```python
from build123d import *

# Parameters (mm, degrees)
F0_R      = 8.5
F1_DEPTH  = 9.5
F3_W      = 16
F3_H      = 14
F4_DEPTH  = 1
F5_W      = 3
F5_H      = 0.5
F6_DEPTH  = 4
F7_R      = 3.5
F8_DEPTH  = 6.5
F9_R      = 3
F10_DEPTH = 13.5
F12_DEPTH = 2


with BuildPart() as f1:
    # F0 (on Front) → F1 (new body)
    with BuildSketch(Plane.XZ):
        Circle(F0_R)
    extrude(amount=-F1_DEPTH)

    # F3 (on offset) → F4 (join)
    with BuildSketch(Plane.XZ.offset(-3.8)):
        with Locations((0, -6)):
            Rectangle(F3_W, F3_H)
    extrude(amount=F4_DEPTH)

    # F5 (on face) → F6 (join)
    with BuildSketch(Plane(origin=(0, 3.8, 0), x_dir=(-1, 0, 0), z_dir=(0, 1, 0))):
        with Locations((0, -12.75)):
            Rectangle(F5_W, F5_H)
        with Locations((-5, -12.75)):
            Rectangle(F5_W, F5_H)
        with Locations((5, -12.75)):
            Rectangle(F5_W, F5_H)
    extrude(amount=F6_DEPTH)

    # F7 (on face) → F8 (join)
    with BuildSketch(Plane.XZ):
        Circle(F7_R)
    extrude(amount=F8_DEPTH)

    # F9 (on face) → F10 (join)
    with BuildSketch(Plane.XZ.offset(6.5)):
        Circle(F9_R)
    extrude(amount=F10_DEPTH)

    # F11 (on face) → F12 (join)
    with BuildSketch(Plane.XZ.offset(6.5)):
        Polygon((5, -2.886751), (5, 2.886751), (0, 5.773503), (-5, 2.886751), (-5, -2.886751), (0, -5.773503), align=None)
    extrude(amount=-F12_DEPTH)


solid = f1.part
```
The model under review builds one solid part; all positions refer to its coordinate system, in mm. A direction names the side the tool comes from. Round coordinates to 2 decimals unless told otherwise and drop trailing zeros. Write each loop counter-clockwise with the first axis right and the second up, starting at its lowest first coordinate (ties: lowest second). Pieces come first, ordered by that corner, then holes. Notation, with made-up numbers: M 22,82 L 76,82 A22 ccw 76,91 Z; hole C 37.5,85.25 d8. An arc over 180 degrees is marked long. Use CSV: the item, a comma, the result in double quotes. Start each with the question number.
(1) For line 1 along Y through (x, z) = (-4.25, 0.5); line 2 along Y through (x, z) = (-5.25, 5.5); line 3 along Y through (x, z) = (6, -9.75), list the stretches that pass through material, from the lowest coordinate up.
(2) Clearance check with flat-ended pins moving along their axes: P1, Ø0.6, axis at y = 5.5, z = -12.5, coming from the +X side; P2, Ø5, axis at x = 0.5, z = -9.5, coming from the -Y side; P3, Ø1.5, axis at x = -6, y = -0.5, coming from the +Z side. State where each tip first meets the part, or that it passes through.
(3) We need section A-A, the plane y = -5. State the section outline as (x, z) points.
(4) We need section C-C, the plane z = 0. State the section outline as (x, y) points, then the cut area to 3 significant figures.
(5) The part is to be moulded in two halves that separate along Z. For faces 6 (the face through (-5, -6, 0)), 7 (the face through (0, 3.8, -10)), 8 (the face through (-3, -13, 0)), say which applies: +Z half, -Z half, draft (parallel to the pull), parting line (faces both ways), or undercut.
(6) We need section D-D, the plane x = 4.5. State the section outline as (y, z) points, then the cut area to 3 significant figures.
(7) Tool access review of faces 1 (the face through (-2.535, -5.514, -4.31)), 2 (the face through (3.233, -2.218, -1.341)), 3 (the face through (0, 2.8, -10)), 4 (the face through (5, -6, 0)), 5 (the face through (-5, 6, -12.5)): name each direction out of +Z, -Z, +X, -X, +Y, -Y from which nothing blocks a thin tool from reaching the whole face with its end or side.
(8) We need section B-B, the plane x = 7.5. State the section outline as (y, z) points, then the cut area to 3 significant figures.
Findings:
1,line 1,"-6.5 to -4.5, 0 to 9.5"
1,line 2,"0 to 9.5"
1,line 3,"2.8 to 3.8"
2,P1,"x = 6.5"
2,P2,"y = 0"
2,P3,"z = 6.53"
3,outline,"M -5,-2.89 L 0,-5.77 L 5,-2.89 L 5,2.89 L 0,5.77 L -5,2.89 Z"
4,outline,"M -8.5,0 L -3.5,0 L -3.5,-4.5 L -5,-4.5 L -5,-6.5 L -3,-6.5 L -3,-20 L 3,-20 L 3,-6.5 L 5,-6.5 L 5,-4.5 L 3.5,-4.5 L 3.5,0 L 8.5,0 L 8.5,9.5 L -8.5,9.5 Z"
4,area,"294 mm^2"
5,face 6,"draft"
5,face 7,"undercut"
5,face 8,"parting line"
6,outline,"M -6.5,-3.18 L -4.5,-3.18 L -4.5,3.18 L -6.5,3.18 Z; M 0,-7.21 L 2.8,-7.21 L 2.8,-13 L 7.8,-13 L 7.8,-12.5 L 3.8,-12.5 L 3.8,-7.21 L 9.5,-7.21 L 9.5,7.21 L 0,7.21 Z"
6,area,"158 mm^2"
7,face 1,"-Z, -X, -Y"
7,face 2,"none"
7,face 3,"-Z, -Y"
7,face 4,"+Z, -Z, +X, -Y"
7,face 5,"+X, -X, +Y"
8,outline,"M 0,-4 L 2.8,-4 L 2.8,-13 L 3.8,-13 L 3.8,-4 L 9.5,-4 L 9.5,4 L 0,4 Z"
8,area,"85.0 mm^2"
